Source: CAD feature listing. Evaluate the final solid. Frame: model axes, mm. Give positions to 0.01 mm unless a question says otherwise; leave off trailing zeros. Write each loop counter-clockwise with the first axis right and the second up, starting at its lowest first coordinate (ties: lowest second). Pieces come first, ordered by that corner, then holes. Notation, with made-up numbers: M 16.25,38.5 L 25.25,38.5 A17 cw 25.25,51.5 Z; hole C 50.25,64 d3. An arc over 180 degrees is marked long. Return JSON: item names as keys, results as strings.
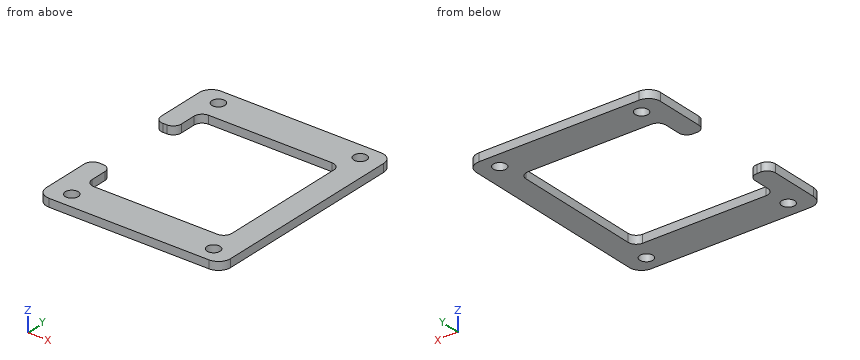
Autodesk Inventor part; units mm, degrees
ref_plane "YZ Plane" through (0, 0, 0) normal (1, 0, 0) x (0, 1, 0)
ref_plane "XZ Plane" through (0, 0, 0) normal (0, 1, 0) x (-1, 0, 0)
ref_plane "XY Plane" through (0, 0, 0) normal (0, 0, 1) x (1, 0, 0)
sketch "Sketch1" plane through (0, 0, 0) normal (0, 0, 1) x (1, 0, 0)
  line L0 (-18.671, 23.6638) -> (26.829, 23.6638)
  line L1 (26.829, 23.6638) -> (26.829, -28.3362)
  line L2 (26.829, -28.3362) -> (-18.671, -28.3362)
  line L3 (-18.671, -28.3362) -> (-18.671, 23.6638)
  point P0 (0, 0)
  dimension "d0" = 52
  dimension "d1" = 45.5
extrude "Extrusion1" add sketch "Sketch1" along normal blind 2
sketch "Sketch2" plane through (0, 0, 2) normal (0, 0, 1) x (1, 0, 0)
  line L0 (-18.671, -28.3362) -> (26.829, -28.3362)
  line L1 (26.829, -28.3362) -> (26.829, 23.6638)
  line L2 (26.829, 23.6638) -> (-18.671, 23.6638)
  point P0 (0, 0)
  point P1 (-13.171, 20.6638)
  point P2 (21.829, 20.6638)
  point P3 (21.829, -25.3362)
  point P4 (-13.171, -25.3362)
  point P5 (23.829, -28.3362)
  point P6 (26.829, -25.3362)
  point P7 (26.829, 20.6638)
  point P8 (23.829, 23.6638)
  dimension "d5" = 35
  dimension "d6" = 35
  dimension "d7" = 46
  dimension "d8" = 3
  dimension "d9" = 3
  dimension "d10" = 5
  dimension "d11" = 5
  dimension "d12" = 3
hole "Hole1" at (-13.171, 20.6638, 2) at (21.829, 20.6638, 2) at (21.829, -25.3362, 2) at (-13.171, -25.3362, 2) direction (0, 0, -1) diameter 3.2 depth 10 tip angle 118
sketch "Sketch3" plane through (0, 0, 2) normal (0, 0, 1) x (1, 0, 0)
  line L0 (-18.671, 23.6638) -> (-18.671, -28.3362)
  line L1 (-18.671, 15.6638) -> (20.829, 15.6638)
  line L2 (20.829, 15.6638) -> (20.829, -20.3362)
  line L3 (20.829, -20.3362) -> (-18.671, -20.3362)
  line L4 (-18.671, -20.3362) -> (-18.671, 15.6638)
  circle A0 centre (-13.171, 20.6638) radius 1.6
  line L5 (26.829, -28.3362) -> (26.829, 23.6638)
  circle A1 centre (-13.171, -25.3362) radius 1.6
  point P0 (0, 0)
  point P1 (26.829, -25.3362)
  point P2 (26.829, 20.6638)
  dimension "d20" = 5
  dimension "d21" = 6
  dimension "d22" = 5
extrude "Extrusion2" cut sketch "Sketch3" against normal blind 2 contours L1 L2 L3 L0
sketch "Sketch4" plane through (0, 0, 2) normal (0, 0, 1) x (1, 0, 0)
  line L0 (-18.671, 15.6638) -> (20.829, 15.6638)
  line L1 (-18.671, 15.6638) -> (-13.671, 15.6638)
  line L2 (-13.671, 15.6638) -> (-13.671, 7.6638)
  line L3 (-13.671, 7.6638) -> (-18.671, 7.6638)
  line L4 (-18.671, 7.6638) -> (-18.671, 15.6638)
  line L5 (-18.671, -20.3362) -> (-18.671, -28.3362)
  line L6 (-18.671, -20.3362) -> (-13.671, -20.3362)
  line L7 (-13.671, -20.3362) -> (-13.671, -12.3362)
  line L8 (-13.671, -12.3362) -> (-18.671, -12.3362)
  line L9 (-18.671, -12.3362) -> (-18.671, -20.3362)
  point P0 (0, 0)
  point P1 (17.829, 15.6638)
  point P2 (-18.671, -25.3362)
  dimension "d27" = 8
  dimension "d28" = 8
  dimension "d29" = 5
extrude "Extrusion3" add sketch "Sketch4" against normal blind 2
fillet "Fillet5" radius 2 4 edges at (-13.671, 7.6638, 1) (-18.671, 7.6638, 1) (-18.671, -12.3362, 1) (-13.671, -12.3362, 1)
sketch "Sketch5" plane through (0, 0, 2) normal (0, 0, 1) x (1, 0, 0)
  line L0 (26.829, 23.6638) -> (-18.671, 23.6638)
  line L1 (-18.671, 23.6638) -> (26.829, 23.6638)
  line L2 (26.829, 23.6638) -> (26.829, 24.6638)
  line L3 (26.829, 24.6638) -> (-18.671, 24.6638)
  line L4 (-18.671, 24.6638) -> (-18.671, 23.6638)
  line L5 (-18.671, -28.3362) -> (26.829, -28.3362)
  line L6 (-18.671, -28.3362) -> (26.829, -28.3362)
  line L7 (26.829, -28.3362) -> (26.829, -29.3362)
  line L8 (26.829, -29.3362) -> (-18.671, -29.3362)
  line L9 (-18.671, -29.3362) -> (-18.671, -28.3362)
  line L10 (26.829, -28.3362) -> (26.829, 23.6638)
  point P0 (0, 0)
  dimension "d37" = 1
  dimension "d38" = 1
extrude "Extrusion4" add sketch "Sketch5" against normal blind 2
fillet "Fillet6" radius 3 4 edges at (-18.671, 24.6638, 1) (26.829, 24.6638, 1) (26.829, -29.3362, 1) (-18.671, -29.3362, 1)
fillet "Fillet7" radius 2 4 edges at (-13.671, 15.6638, 1) (20.829, 15.6638, 1) (20.829, -20.3362, 1) (-13.671, -20.3362, 1)
properties part number "wood_supp"
1) Cut plane C-C, the plane z = 1.35. Return the cut outline in (x, y).
Numbers:
{"outline": "M -18.67,-26.34 A3 ccw -15.67,-29.34 L 23.83,-29.34 A3 ccw 26.83,-26.34 L 26.83,21.66 A3 ccw 23.83,24.66 L -15.67,24.66 A3 ccw -18.67,21.66 L -18.67,9.66 A2 ccw -16.67,7.66 L -15.67,7.66 A2 ccw -13.67,9.66 L -13.67,13.66 A2 cw -11.67,15.66 L 18.83,15.66 A2 cw 20.83,13.66 L 20.83,-18.34 A2 cw 18.83,-20.34 L -11.67,-20.34 A2 cw -13.67,-18.34 L -13.67,-14.34 A2 ccw -15.67,-12.34 L -16.67,-12.34 A2 ccw -18.67,-14.34 Z; hole C -13.17,-25.34 d3.2; hole C -13.17,20.66 d3.2; hole C 21.83,-25.34 d3.2; hole C 21.83,20.66 d3.2"}
2) Cut plane B-B, the plane y = -25. Return the cut outline in (x, z).
Numbers:
{"outline": "M -18.67,0 L -14.74,0 L -14.74,2 L -18.67,2 Z; M -11.61,0 L 20.26,0 L 20.26,2 L -11.61,2 Z; M 23.39,0 L 26.83,0 L 26.83,2 L 23.39,2 Z"}
3) Cut plane A-A, the plane x = 4. Return the cut outline in (y, z), then the cut area to 3 significant figures.
Numbers:
{"outline": "M -29.34,0 L -20.34,0 L -20.34,2 L -29.34,2 Z; M 15.66,0 L 24.66,0 L 24.66,2 L 15.66,2 Z", "area": "36.0 mm²"}
4) Cut plane D-D, the plane y = -19.5. Return the cut outline in (x, z), then the cut area to 3 significant figures.
Numbers:
{"outline": "M -18.67,0 L -13.3,0 L -13.3,2 L -18.67,2 Z; M 20.46,0 L 26.83,0 L 26.83,2 L 20.46,2 Z", "area": "23.5 mm²"}
5) Line query: line 1 (X direction, y = -16.5, z = 1.05); line 2 (Y direction, x = -3.5, z = 0.85); line 3 (X direction, y = 21.5, z = 0.8). Output: solid intervals per line, ascending. Write a range as [from, to].
Numbers:
{"line 1": "x = [-18.67, -13.67], [20.83, 26.83]", "line 2": "y = [-29.34, -20.34], [15.66, 24.66]", "line 3": "x = [-18.67, -14.54], [-11.81, 20.46], [23.19, 26.83]"}
6) Contact query for flat-ended pins moving along their axis: pin 1 Ø0.5 at (x, z) = (-16.5, 1.5) entering from -Y; pin 2 Ø0.6 at (y, z) = (-8, 1) entering from -X; pin 3 Ø2.5 at (x, y) = (21.83, -25.34) entering from +Z. Output: stop coordinate, or through.
Numbers:
{"pin 1": "stops at y = -29.28", "pin 2": "stops at x = 20.83", "pin 3": "passes through"}
